Verification items for the finished model (mm, model axes). Face numbers are marked on the shaded views. A direction names the side the tool comes from. Give positions to 0.01 mm unless a question says otherwise; leave off trailing zeros. Loops run counter-clockwise (first coordinate to the right, second up) from the corner with the lowest first, then second, coordinate; pieces in that order, holes last. Notation, with made-up numbers: (57.5, 52.25) - (87.5, 52.25) arc R29 ccw to (87.5, 89.25) - close; hole circle Ø2 at (-5.5, 38). An arc over 180 degrees is marked (long way). One line per question, with ' | ' between items. Start each with the question number.
1. Section check B-B, the plane y = -10. Enter the section's corners in (x, z).
2. Mould release check, pull along Z, two halves, no side actions. Record for the marked faces 1, 2 and 3: +Z half, -Z half, draft (parallel to the pull), parting line (faces both ways), or undercut.
3. Section check D-D, the plane x = -6.75. Enter the section's corners in (y, z), then the cut area to 3 significant figures.
4. Depth check by flat-ended pin: pin 1 Ø6.5 at (x, z) = (1.5, -0.5) entering from -Y; pin 2 Ø1 at (x, z) = (0, 7) entering from -Y. Enter the tip coordinate at first touch or a pass-through.
5. Thickness scan on line 1 along Z through (x, y) = (6.5, -13.25); line 2 along X through (y, z) = (-14.5, -1.5); line 3 along Y through (x, z) = (6.75, -0.75). Record the ranges inside material, lowest first. Write a range as from..to.
6. Section check C-C, the plane z = 0.5. Enter the section's corners in (x, y).
7. Tool access check on the marked faces 4 and 5. Record the directions out of +Z, -Z, +X, -X, +Y, -Y that give a thin tool (end or side, any length) a straight path to the whole face; none if there is none.
8. Section check A-A, the plane x = 1. Enter the section's corners in (y, z), then the cut area to 3 significant figures.
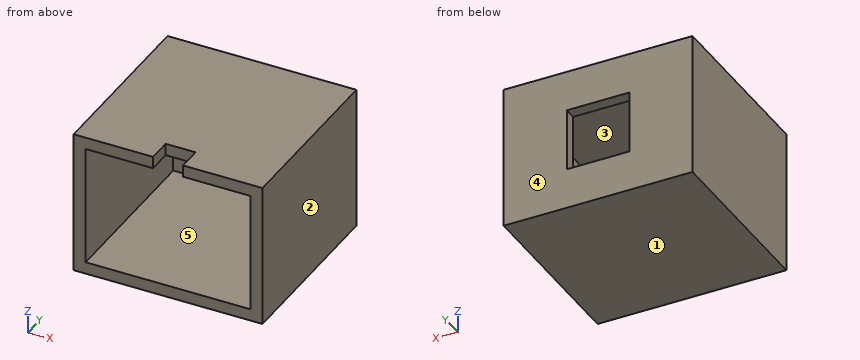
Autodesk Inventor part; units mm, degrees
ref_plane "YZ Plane" through (0, 0, 0) normal (1, 0, 0) x (0, 1, 0)
ref_plane "XZ Plane" through (0, 0, 0) normal (0, 1, 0) x (-1, 0, 0)
ref_plane "XY Plane" through (0, 0, 0) normal (0, 0, 1) x (1, 0, 0)
sketch "Sketch1" plane through (0, 0, 0) normal (0, 1, 0) x (-1, 0, 0)
  line L0 (8.7312, 6.35) -> (-8.7313, 6.35)
  line L1 (-8.7313, 6.35) -> (-8.7312, -6.35)
  line L2 (-8.7312, -6.35) -> (8.7313, -6.35)
  line L3 (8.7313, -6.35) -> (8.7312, 6.35)
  line L4 (3.302, -3.302) -> (-3.302, -3.302)
  line L5 (-3.302, -3.302) -> (-3.302, 3.302)
  line L6 (-3.302, 3.302) -> (3.302, 3.302)
  line L7 (3.302, 3.302) -> (3.302, -3.302)
  point P0 (0, 0)
  dimension "d0" = 12.7
  dimension "d1" = 17.4625
  dimension "d2" = 6.35
  dimension "d3" = 8.7312
  dimension "d16" = 6.604
  dimension "d17" = 6.604
  dimension "d18" = 3.302
  dimension "d19" = 3.302
extrude "Extrusion1" add sketch "Sketch1" along normal blind 1.27
sketch "Sketch2" plane through (0, 1.27, 0) normal (0, 1, 0) x (1, 0, 0)
  line L0 (8.7313, -6.35) -> (8.7312, 6.35)
  line L1 (8.7312, 6.35) -> (-8.7313, 6.35)
  line L2 (-8.7313, 6.35) -> (-8.7312, -6.35)
  line L3 (-8.7312, -6.35) -> (8.7313, -6.35)
  line L4 (-10.0012, -7.62) -> (-10.0013, 7.62)
  line L5 (-10.0013, 7.62) -> (10.0013, 7.62)
  line L6 (10.0013, 7.62) -> (10.0013, -7.62)
  line L7 (10.0013, -7.62) -> (-10.0012, -7.62)
  point P0 (0, 0)
  dimension "d7" = 1.27
extrude "Extrusion2" add sketch "Sketch2" against normal blind 19.05
sketch "Sketch3" plane through (-10.0012, 1.27, 7.62) normal (0, 0, 1) x (1, 0, 0)
  line L0 (0, 0) -> (20.0025, 0)
  line L1 (0, 0) -> (0, -19.05)
  line L2 (20.0025, -19.05) -> (0, -19.05)
  line L3 (20.0025, 0) -> (20.0025, -19.05)
  line L4 (0, -19.05) -> (20.0025, -19.05)
  line L5 (8.4138, -19.05) -> (11.5888, -19.05)
  line L6 (11.5888, -19.05) -> (11.5887, -16.51)
  line L7 (11.5887, -16.51) -> (8.4138, -16.51)
  line L8 (8.4138, -16.51) -> (8.4138, -19.05)
  point P0 (10.0012, -1.27)
  point P1 (10.0012, -16.51)
  dimension "d10" = 3.175
  dimension "d11" = 20.0025
  dimension "d12" = 10.0013
  dimension "d13" = 2.54
extrude "Extrusion3" cut sketch "Sketch3" against normal blind 3.81 contours L8 L7 L6 L2
properties part number "button_holder"
Results list:
1) outline: (-10, -7.62) - (10, -7.62) - (10, 7.62) - (-10, 7.62) - close; hole (-8.73, -6.35) - (8.73, -6.35) - (8.73, 6.35) - (-8.73, 6.35) - close
2) face 1: -Z half | face 2: draft | face 3: undercut
3) outline: (-17.78, -7.62) - (1.27, -7.62) - (1.27, 7.62) - (-17.78, 7.62) - (-17.78, 6.35) - (0, 6.35) - (0, -6.35) - (-17.78, -6.35) - close | area: 64.5 mm²
4) pin 1: y = 0 | pin 2: y = -15.24
5) line 1: -7.62..-6.35, 6.35..7.62 | line 2: -10..-8.73, 8.73..10 | line 3: 0..1.27
6) outline: (-10, -17.78) - (-8.73, -17.78) - (-8.73, 0) - (-3.3, 0) - (-3.3, 1.27) - (-10, 1.27) - close; (3.3, 0) - (8.73, 0) - (8.73, -17.78) - (10, -17.78) - (10, 1.27) - (3.3, 1.27) - close
7) face 4: +Z, -Z, +X, -X, +Y | face 5: -Y
8) outline: (-17.78, -7.62) - (1.27, -7.62) - (1.27, -3.3) - (0, -3.3) - (0, -6.35) - (-17.78, -6.35) - close; (-15.24, 6.35) - (0, 6.35) - (0, 3.3) - (1.27, 3.3) - (1.27, 7.62) - (-15.24, 7.62) - close | area: 52.9 mm²
